The listing builds one solid part. Answer for the finished solid, in the listing's coordinates (mm). Coordinates: 2 decimals unless noted, no trailing zeros. Write each loop counter-clockwise with the first axis right and the second up, starting at its lowest first coordinate (ties: lowest second). Pieces come first, ordered by that corner, then holes.
Autodesk Inventor part; units mm, degrees
ref_plane "YZ Plane" through (0, 0, 0) normal (1, 0, 0) x (0, 1, 0)
ref_plane "XZ Plane" through (0, 0, 0) normal (0, 1, 0) x (-1, 0, 0)
ref_plane "XY Plane" through (0, 0, 0) normal (0, 0, 1) x (1, 0, 0)
sketch "Sketch1" plane through (0, 0, 0) normal (0, 0, 1) x (1, 0, 0)
  line L0 (0, 0) -> (304.8, 0)
  line L1 (304.8, 0) -> (304.8, 330.2)
  line L2 (304.8, 330.2) -> (0, 330.2)
  line L3 (0, 330.2) -> (0, 0)
  dimension "d0" = 304.8
  dimension "d1" = 330.2
extrude "Extrusion1" add sketch "Sketch1" along normal blind 6.35
sketch "Sketch2" plane through (0, 0, 0) normal (0, 0, -1) x (-1, 0, 0)
  line L0 (-323.0002, 172.6) -> (-260.0002, 172.6)
  line L1 (-323.0002, 132.2) -> (-260.0002, 132.2)
  line L2 (-246.7514, 152.4) -> (-364.8335, 152.4)
  line L3 (-304.8, 0) -> (-304.8, 330.2)
  line L4 (-304.8, 172.6) -> (-260.0002, 172.6)
  line L5 (-260.0002, 172.6) -> (-260.0002, 132.2)
  line L6 (-260.0002, 132.2) -> (-304.8, 132.2)
  line L7 (-304.8, 132.2) -> (-304.8, 172.6)
  point P0 (0, 0)
  dimension "d4" = 20.2
  dimension "d5" = 20.2
extrude "Extrusion2" cut sketch "Sketch2" against normal blind 25.4
ref_plane "Work Plane1" through (152.4, 330.2, 6.35) normal (1, 0, 0) x (0, 0, -1)
mirror "Mirror1" about plane through (152.4, 330.2, 6.35) normal (1, 0, 0) of "Extrusion2"
sketch "Sketch3" plane through (0, 0, 0) normal (0, 0, -1) x (-1, 0, 0)
  circle A0 centre (-203.2502, 165.1) radius 2.0193
  circle A1 centre (-247.7002, 165.1) radius 2.0193
  circle A2 centre (-247.7002, 139.7) radius 2.0193
  circle A3 centre (-203.2502, 139.7) radius 2.0193
  circle A4 centre (-101.5498, 165.1) radius 2.0193
  circle A5 centre (-101.5498, 139.7) radius 2.0193
  circle A6 centre (-57.0998, 165.1) radius 2.0193
  circle A7 centre (-57.0998, 139.7) radius 2.0193
  point P0 (0, 0)
hole "Hole1" at (247.7002, 165.1, 0) at (203.2502, 165.1, 0) at (203.2502, 139.7, 0) at (247.7002, 139.7, 0) at (101.5498, 165.1, 0) at (101.5498, 139.7, 0) at (57.0998, 139.7, 0) at (57.0998, 165.1, 0) direction (0, 0, 1) diameter 6.35 depth 25.4 tip angle 118
sketch "Sketch4" plane through (0, 0, 0) normal (0, 0, -1) x (-1, 0, 0)
  circle A0 centre (-292.1, 317.5) radius 1.27
  circle A1 centre (-292.1, 266.7) radius 1.27
  circle A2 centre (-292.1, 241.3) radius 1.27
  circle A3 centre (-292.1, 292.1) radius 1.27
  line L0 (-302.26, 228.6) -> (-281.94, 228.6)
  line L1 (-281.94, 228.6) -> (-281.94, 330.2)
  line L2 (-302.26, 330.2) -> (-281.94, 330.2)
  line L3 (-302.26, 228.6) -> (-302.26, 330.2)
  line L4 (-281.94, 101.6) -> (-302.26, 101.6)
  line L5 (-302.26, 0) -> (-302.26, 101.6)
  line L6 (-281.94, 0) -> (-302.26, 0)
  line L7 (-281.94, 0) -> (-281.94, 101.6)
  circle A4 centre (-292.1, 63.5) radius 1.27
  circle A5 centre (-292.1, 12.7) radius 1.27
  circle A6 centre (-292.1, 38.1) radius 1.27
  circle A7 centre (-292.1, 88.9) radius 1.27
  point P0 (0, 0)
hole "Hole2" at (292.1, 317.5, 0) at (292.1, 292.1, 0) at (292.1, 266.7, 0) at (292.1, 241.3, 0) at (292.1, 88.9, 0) at (292.1, 63.5, 0) at (292.1, 38.1, 0) at (292.1, 12.7, 0) direction (0, 0, 1) diameter 1.778 depth 19.05 tip angle 118
mirror "Mirror2" about plane through (152.4, 330.2, 6.35) normal (1, 0, 0) of "Hole2"
sketch "Sketch5" plane through (0, 0, 0) normal (0, 0, -1) x (-1, 0, 0)
  circle A0 centre (-124.5248, 165.1) radius 1.27
  circle A1 centre (-124.5248, 215.9) radius 1.27
  circle A2 centre (-124.5248, 266.7) radius 1.27
  circle A3 centre (-124.5248, 317.5) radius 1.27
  circle A4 centre (-124.5248, 292.1) radius 1.27
  circle A5 centre (-124.5248, 241.3) radius 1.27
  circle A6 centre (-124.5248, 190.5) radius 1.27
  circle A7 centre (-124.5248, 139.7) radius 1.27
  line L0 (-114.3648, 330.2) -> (-134.6848, 330.2)
  line L1 (-114.3648, 330.2) -> (-114.3648, 127)
  line L2 (-134.6848, 127) -> (-114.3648, 127)
  line L3 (-134.6848, 330.2) -> (-134.6848, 127)
  circle A8 centre (-180.2752, 165.1) radius 1.27
  circle A9 centre (-180.2752, 215.9) radius 1.27
  circle A10 centre (-180.2752, 266.7) radius 1.27
  circle A11 centre (-180.2752, 317.5) radius 1.27
  circle A12 centre (-180.2752, 292.1) radius 1.27
  circle A13 centre (-180.2752, 241.3) radius 1.27
  circle A14 centre (-180.2752, 190.5) radius 1.27
  circle A15 centre (-180.2752, 139.7) radius 1.27
  line L4 (-170.1152, 330.2) -> (-190.4352, 330.2)
  line L5 (-170.1152, 330.2) -> (-170.1152, 127)
  line L6 (-190.4352, 127) -> (-170.1152, 127)
  line L7 (-190.4352, 330.2) -> (-190.4352, 127)
  point P0 (0, 0)
hole "Hole3" at (180.2752, 139.7, 0) at (124.5248, 139.7, 0) at (124.5248, 165.1, 0) at (180.2752, 165.1, 0) at (180.2752, 190.5, 0) at (124.5248, 190.5, 0) at (124.5248, 215.9, 0) at (180.2752, 215.9, 0) at (124.5248, 241.3, 0) at (180.2752, 241.3, 0) at (180.2752, 266.7, 0) at (124.5248, 266.7, 0) at (124.5248, 292.1, 0) at (180.2752, 292.1, 0) at (124.5248, 317.5, 0) at (180.2752, 317.5, 0) direction (0, 0, 1) diameter 4.4958 depth 19.05 tip angle 118
sketch "Sketch6" plane through (0, 0, 0) normal (0, 0, -1) x (-1, 0, 0)
  line L0 (-165.1, 175.9057) -> (-165.1, -141.7236)
  line L1 (-137.2248, 330.2) -> (-137.2248, 127)
  line L2 (-167.5752, 330.2) -> (-167.5752, 127)
  line L3 (-139.7, 175.9057) -> (-139.7, -141.7236)
  line L4 (-167.5752, 330.2) -> (-167.5752, 127)
  line L5 (-167.5752, 127) -> (-137.2248, 127)
  line L6 (-137.2248, 127) -> (-137.2248, 215.9)
  line L7 (-137.2248, 215.9) -> (-167.5752, 215.9)
  line L8 (-167.5752, 215.9) -> (-167.5752, 127)
  line L9 (-167.5752, 127) -> (-137.2248, 127)
  line L10 (-137.2248, 127) -> (-137.2248, 76.2)
  line L11 (-137.2248, 76.2) -> (-167.5752, 76.2)
  line L12 (-167.5752, 76.2) -> (-167.5752, 127)
  point P0 (0, 0)
  dimension "d29" = 88.9
  dimension "d31" = 50.8
extrude "Extrusion3" cut sketch "Sketch6" against normal blind 25.4
sketch "Sketch8" plane through (0, 0, 0) normal (0, 0, -1) x (-1, 0, 0)
  circle A0 centre (-1186.1371, 107.95) radius 1.27
  circle A1 centre (-1211.5371, 107.95) radius 1.27
  circle A2 centre (-1236.9371, 107.95) radius 1.27
  circle A3 centre (-1262.3371, 107.95) radius 1.27
  circle A4 centre (-1287.7371, 107.95) radius 1.27
  circle A5 centre (-1313.1371, 107.95) radius 1.27
  circle A6 centre (-1338.5371, 107.95) radius 1.27
  circle A7 centre (-1363.9371, 107.95) radius 1.27
  circle A8 centre (-1389.3371, 107.95) radius 1.27
  circle A9 centre (-1414.7371, 107.95) radius 1.27
  point P0 (0, 0)
hole "Hole4" at (1186.1371, 107.95, 0) at (1211.5371, 107.95, 0) at (1236.9371, 107.95, 0) at (1262.3371, 107.95, 0) at (1287.7371, 107.95, 0) at (1313.1371, 107.95, 0) at (1338.5371, 107.95, 0) at (1363.9371, 107.95, 0) at (1389.3371, 107.95, 0) at (1414.7371, 107.95, 0) direction (0, 0, 1) diameter 4.4958 depth 19.05 tip angle 118
equation "\"d4\" = d5"
properties part number "Piv Pannel 2" material "Polycarbonate, Clear"
1. Section A-A on x = 40.5 is taken. Give the vertices of the cut face in (y, z), then the cut area to 3 significant figures.
Results found:
outline: (0, 0) - (132.2, 0) - (132.2, 6.35) - (0, 6.35) - close; (172.6, 0) - (330.2, 0) - (330.2, 6.35) - (172.6, 6.35) - close
area: 1,840 mm2
2. Find the intervals of material crossed by L1, parallel to Y at x = 204, z = 5; L2, parallel to X at y = 241.3, z = 4.75; L3, parallel to X at y = 38.1, z = 2, in increasing order.
Results found:
L1: y = 0 to 136.61, 142.79 to 162.01, 168.19 to 330.2
L2: x = 0 to 11.81, 13.59 to 122.28, 126.77 to 178.03, 182.52 to 291.21, 292.99 to 304.8
L3: x = 0 to 11.81, 13.59 to 291.21, 292.99 to 304.8
3. Section C-C on z = 4.75 is taken. State how many separate pieces and enclosed holes the cut face has, then the cut area to 3 significant figures.
Results found:
separate pieces: 1
enclosed holes: 41
area: 92,200 mm2
4. A flat-ended cylindrical pin translates along its axis: P1, Ø3, axis at x = 292.1, y = 63.5, coming from the -Z side. Find the tip coordinate at first contact, or state that the pin passes through.
Results found:
P1: stops at z = 0
5. Section B-B on y = 197 is taken. Give the vertices of the cut face in (x, z).
Results found:
outline: (0, 0) - (137.22, 0) - (137.22, 6.35) - (0, 6.35) - close; (167.58, 0) - (304.8, 0) - (304.8, 6.35) - (167.58, 6.35) - close
